from build123d import *

# Parameters (mm, degrees)
F0_R     = 3.425
F0_W     = 60
F0_H     = 60
F1_DEPTH = 5
F2_DEPTH = 9.5


with BuildPart() as f1:
    # F0 (on Top) → F1 (new body)
    with BuildSketch(Plane.XY):
        with BuildLine():
            Line((-25, -50), (25, -50))
            ThreePointArc((25, -50), (42.67767, -42.67767), (50, -25))
            Line((50, -25), (50, 25))
            ThreePointArc((50, 25), (42.67767, 42.67767), (25, 50))
            Line((25, 50), (-25, 50))
            ThreePointArc((-25, 50), (-42.67767, 42.67767), (-50, 25))
            Line((-50, 25), (-50, -25))
            ThreePointArc((-50, -25), (-42.67767, -42.67767), (-25, -50))
        make_face()
        with Locations((-40.562063, 0)):
            Circle(F0_R, mode=Mode.SUBTRACT)
        Rectangle(F0_W, F0_H, mode=Mode.SUBTRACT)
        with Locations((40.562063, 0)):
            Circle(F0_R, mode=Mode.SUBTRACT)
    extrude(amount=F1_DEPTH)

    # F0 (on Top) → F2 (join)
    with BuildSketch(Plane.XY):
        with Locations((-40.562063, 0)):
            Circle(F0_R)
        with Locations((40.562063, 0)):
            Circle(F0_R)
    extrude(amount=F2_DEPTH)


solid = f1.part
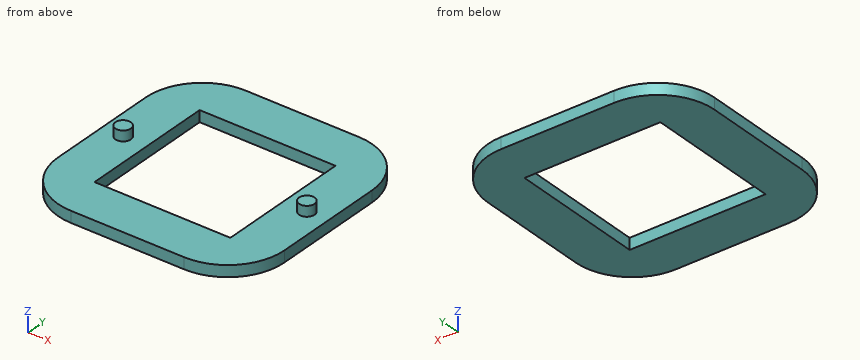
Part model, mm, in its own coordinate system. Coordinates: 2 decimals unless noted, no trailing zeros. Loops run counter-clockwise (first coordinate to the right, second up) from the corner with the lowest first, then second, coordinate; pieces in that order, holes last. Notation, with made-up numbers: (87.25, 15.5) - (96.25, 15.5) arc R31 cw to (96.25, 52.5) - close; hole circle Ø11 at (5.25, 39.25). An arc over 180 degrees is marked (long way). Write each question's results on one line, items separated by ' | '. Start each with the question number.
Q1. Slice it at C-C on z = 1.25. Give the cut face in (x, y).
Q2. Drop flat-ended pins along their axis: pin 1 Ø1.5 at (x, z) = (-32.5, 5.5) entering from +Y; pin 2 Ø6 at (x, y) = (-25.5, -1) entering from +Z; pin 3 Ø1.5 at (x, y) = (30.5, -22.5) entering from +Z. Give the stop position or say it passes through.
Q3. Slice it at B-B on x = 7. Give the cut face in (y, z).
Q4. Slice it at A-A on y = 0. Give the cut face in (x, z), and give its area (3 significant figures).
Q5. Probe line 1 along Y through (x, z) = (-10, 1.25); line 2 along Z through (x, y) = (-35, -27). List the from-to ranges inside material, lowest first.
Answer:
1) outline: (-50, -25) arc R25 ccw to (-25, -50) - (25, -50) arc R25 ccw to (50, -25) - (50, 25) arc R25 ccw to (25, 50) - (-25, 50) arc R25 ccw to (-50, 25) - close; hole (-30, -30) - (30, -30) - (30, 30) - (-30, 30) - close
2) pin 1: stops at y = 49.02 | pin 2: passes through | pin 3: stops at z = 5
3) outline: (-50, 0) - (-30, 0) - (-30, 5) - (-50, 5) - close; (30, 0) - (50, 0) - (50, 5) - (30, 5) - close
4) outline: (-50, 0) - (-30, 0) - (-30, 5) - (-37.14, 5) - (-37.14, 9.5) - (-43.99, 9.5) - (-43.99, 5) - (-50, 5) - close; (30, 0) - (50, 0) - (50, 5) - (43.99, 5) - (43.99, 9.5) - (37.14, 9.5) - (37.14, 5) - (30, 5) - close | area: 262 mm2
5) line 1: y = -50 to -30, 30 to 50 | line 2: z = 0 to 5
